Check sheet for the modelled part. Datum: model origin and axes. Units: mm. A direction names the side the tool comes from. Give positions to 0.01 mm unless a question says otherwise; leave off trailing zeros. Order: outer loops, then holes, each group sorted by start corner. A loop starts at its lowest first (then second) coordinate and runs counter-clockwise, first axis right, second up.
Item 1: Release check for a two-part mould opening along Z. For faces 1 (the flat face through (-8.8, -12.004, -3.6)), 2 (the cylindrical face through (3.01, 7.22, 1.52)), 3 (the flat face through (-3, -3, 3)) record: released by +Z, released by -Z, zero draft, split by the parting line, or undercut.
Item 2: Material ranges on line 1 along X through (y, z) = (-12.6, -5); line 2 along Z through (x, y) = (8.5, 11); line 3 along Y through (x, z) = (-11, -2.25), recorded low to high.
Item 3: Sectioned sample at B-B on x = -1. Record the boundary of the cut face in (y, z).
Item 4: Sectioned sample at A-A on y = 2.5. Record the boundary of the cut face in (x, z), and give its area (3 significant figures).
Item 5: Gauge pin test, flat ends, axial feed: P1, Ø3, axis at y = 8, z = 0.5, coming from the +X side; P2, Ø4, axis at x = 6.81, z = -5, coming from the +Y side; P3, Ø4.5, axis at x = -7, z = -4, coming from the +Y side. Record the tip position at first contact, or that the pin passes through.
Item 6: Access from +Z, -Z, +X, -X, +Y, -Y to the whole of each face (thin tool, end or side, straight path). Record for faces 4 (the flat face through (-10.313, -11, -5)), 5 (the flat face through (-3, -3, 0)), 6 (the flat face through (0, -12, -10)).
Item 7: Sectioned sample at C-C on z = -5. Record the boundary of the cut face in (x, y).
Item 8: Sectioned sample at D-D on x = 6.25. Record the boundary of the cut face in (y, z), and give its area (3 significant figures).
from build123d import *

# Parameters (mm, degrees)
SKETCH_1_W           = 25
SKETCH_1_H           = 27
EXTRUDE_1_DEPTH      = 3
SKETCH_2_W           = 25
SKETCH_2_H           = 2.996002967
EXTRUDE_2_DEPTH      = 10
SKETCH_3_R           = 5.6
CUT_EXTRUDE_1_DEPTH  = 10
FILLET_1_R           = 10
SKETCH_4_R           = 1.75
CUT_EXTRUDE_2_DEPTH  = 10
FILLET_2_R           = 1
CUT_EXTRUDE_3_DEPTH  = 1.5
SKETCH_6_R           = 1.5
CUT_EXTRUDE_10_DEPTH = 23.527760652


with BuildPart() as part:
    # Эскиз1 → Бобышка-Вытянуть1 (new body)
    with BuildSketch(Plane.XY):
        Rectangle(SKETCH_1_W, SKETCH_1_H)
    extrude(amount=EXTRUDE_1_DEPTH)

    # Эскиз2 → Бобышка-Вытянуть2 (add)
    with BuildSketch(Plane(origin=(0, 0, 0), x_dir=(-1, 0, 0), z_dir=(0, 0, -1))):
        with Locations((0, -12.001998517)):
            Rectangle(SKETCH_2_W, SKETCH_2_H)
    extrude(amount=EXTRUDE_2_DEPTH)

    # Эскиз3 → Вырез-Вытянуть1 (cut)
    with BuildSketch(Plane.XY.offset(3)):
        with Locations((0, 2.5)):
            Circle(SKETCH_3_R)
    extrude(amount=-CUT_EXTRUDE_1_DEPTH, mode=Mode.SUBTRACT)

    # Скругление1
    fillet_1_edges = [part.edges().sort_by_distance(p)[0] for p in [
        (-12.5, 13.5, 1.5),
        (12.5, 13.5, 1.5),
    ]]
    fillet(fillet_1_edges, radius=FILLET_1_R)

    # Эскиз4 → Вырез-Вытянуть2 (cut)
    with BuildSketch(Plane.XZ.offset(13.5)):
        with Locations(Location((-7.513385328, -5, 0), (0, 0, 270))):
            Circle(SKETCH_4_R)
        with Locations(Location((6.812780265, -5, 0), (0, 0, 270))):
            Circle(SKETCH_4_R)
    extrude(amount=-CUT_EXTRUDE_2_DEPTH, mode=Mode.SUBTRACT)

    # Скругление2
    fillet_2_edges = [part.edges().sort_by_distance(p)[0] for p in [
        (0, -10.503997033, 0),
    ]]
    fillet(fillet_2_edges, radius=FILLET_2_R)

    # Эскиз5 → Вырез-Вытянуть3 (cut)
    with BuildSketch(Plane(origin=(0, -10.503997033, 0), x_dir=(1, 0, 0), z_dir=(0, 1, 0))):
        Polygon((9.612780265, 3.383419246), (9.612780265, 6.616580754), (6.812780265, 8.233161507), (4.012780265, 6.616580754), (4.012780265, 3.383419246), (6.812780265, 1.766838493), align=None)
        Polygon((-4.713385328, 3.383419246), (-4.713385328, 6.616580754), (-7.513385328, 8.233161507), (-10.313385328, 6.616580754), (-10.313385328, 3.383419246), (-7.513385328, 1.766838493), align=None)
    extrude(amount=-CUT_EXTRUDE_3_DEPTH, mode=Mode.SUBTRACT)

    # Эскиз6 → Вырез-Вытянуть10 (cut, through all)
    with BuildSketch(Plane.XY.offset(3)):
        with Locations((-10, 2.5)):
            Circle(SKETCH_6_R)
        with Locations((10, 2.5)):
            Circle(SKETCH_6_R)
    extrude(amount=-CUT_EXTRUDE_10_DEPTH, mode=Mode.SUBTRACT)


solid = part.part
Report:
1. face 1: undercut
1. face 2: zero draft
1. face 3: released by +Z
2. line 1: x = -12.5 to -9.26, -5.76 to 5.06, 8.56 to 12.5
2. line 2: z = 0 to 3
2. line 3: y = -13.5 to -10.5
3. outline: (-13.5, -10) - (-10.5, -10) - (-10.5, -1) arc R1 cw to (-9.5, 0) - (-3.01, 0) - (-3.01, 3) - (-13.5, 3) - close; (8.01, 0) - (13.5, 0) - (13.5, 3) - (8.01, 3) - close
4. outline: (-12.5, 0) - (-11.5, 0) - (-11.5, 3) - (-12.5, 3) - close; (-8.5, 0) - (-5.6, 0) - (-5.6, 3) - (-8.5, 3) - close; (5.6, 0) - (8.5, 0) - (8.5, 3) - (5.6, 3) - close; (11.5, 0) - (12.5, 0) - (12.5, 3) - (11.5, 3) - close
4. area: 23.4 mm2
5. P1: stops at x = 12.04
5. P2: stops at y = -12
5. P3: stops at y = -10.5
6. face 4: +Y
6. face 5: -Z, +X, -X, +Y
6. face 6: -Z, +X, -X, +Y, -Y
7. outline: (-12.5, -13.5) - (-9.26, -13.5) - (-9.26, -12) - (-10.31, -12) - (-10.31, -10.5) - (-12.5, -10.5) - close; (-5.76, -13.5) - (5.06, -13.5) - (5.06, -12) - (4.01, -12) - (4.01, -10.5) - (-4.71, -10.5) - (-4.71, -12) - (-5.76, -12) - close; (8.56, -13.5) - (12.5, -13.5) - (12.5, -10.5) - (9.61, -10.5) - (9.61, -12) - (8.56, -12) - close
8. outline: (-13.5, -10) - (-10.5, -10) - (-10.5, -7.91) - (-12, -7.91) - (-12, -6.66) - (-13.5, -6.66) - close; (-13.5, -3.34) - (-12, -3.34) - (-12, -2.09) - (-10.5, -2.09) - (-10.5, -1) arc R1 cw to (-9.5, 0) - (12.77, 0) - (12.77, 3) - (-13.5, 3) - close
8. area: 95.3 mm2
